Autodesk Inventor part; units mm, degrees
ref_plane "YZ Plane" through (0, 0, 0) normal (1, 0, 0) x (0, 1, 0)
ref_plane "XZ Plane" through (0, 0, 0) normal (0, 1, 0) x (-1, 0, 0)
ref_plane "XY Plane" through (0, 0, 0) normal (0, 0, 1) x (1, 0, 0)
sketch "Sketch1" plane through (0, 0, 0) normal (0, 1, 0) x (-1, 0, 0)
  arc A0 (-31.1503, 12.1688) -> (-35.4003, 7.9188) centre (-35.4003, 12.1688) ccw
  line L0 (-35.4003, 16.4188) -> (-35.4003, -2.5812)
  line L1 (-39.6503, 12.1688) -> (-31.1503, 12.1688)
  line L2 (-39.6503, -2.5812) -> (-39.6503, 12.1688)
  line L3 (-35.4003, 12.1688) -> (-26.4003, 12.1688)
  line L4 (-35.4003, 16.4188) -> (-26.4003, 16.4188)
  line L5 (-26.4003, 16.4188) -> (-26.4003, 7.9188)
  line L6 (-26.4003, 7.9188) -> (-35.4003, 7.9188)
  line L7 (-35.4003, 7.9188) -> (-35.4003, 16.4188)
  arc A1 (-35.4003, 7.9188) -> (-31.1503, 12.1688) centre (-35.4003, 12.1688) ccw
  line L8 (-35.4003, -2.5812) -> (-39.6503, -2.5812)
  point P0 (0, 0)
  dimension "d0" = 8.5
  dimension "d3" = 19
  dimension "d4" = 9
extrude "Extrusion2" add sketch "Sketch1" along normal blind 3
extrude "Extrusion3" add sketch "Sketch1" along normal blind 9 contours L1 L0 A0 | A1 L0 L1 | L0 L1 A0 | L0 A0 L1
sketch "Sketch2" plane through (35.4003, 9, 12.1688) normal (0, 1, 0) x (1, 0, 0)
  circle A0 centre (0, 0) radius 4.25
  circle A1 centre (0, 0) radius 4.25
  point P0 (-35.4003, 12.1688)
hole "Hole1" at (35.4003, 9, 12.1688) direction (0, -1, 0) diameter 2.4384 end through all
mirror "Mirror1" about plane through (39.6503, 0, -2.5812) normal (0, 0, -1) of "Extrusion2", "Extrusion3", "Hole1"
mirror "Mirror2" about plane through (26.4003, 0, -13.0812) normal (-1, 0, 0) of "Extrusion2", "Extrusion3", "Hole1", "Mirror1"
properties part number "Spacer"
Verification items for the finished model (mm, model axes). A direction names the side the tool comes from. Coordinates: 2 decimals unless noted, no trailing zeros. Order: outer loops, then holes, each group sorted by start corner. A loop starts at its lowest first (then second) coordinate and runs counter-clockwise, first axis right, second up. Notation, with made-up numbers: M 44,-28.75 L 88,-28.75 A32 cw 88,10.25 Z; hole C 58,21.5 d10. An arc over 180 degrees is marked long. One line per item, written item: value. Start each with the question number.
Item 1: Sectioned sample at C-C (x = 24). Enter the section's corners in (y, z).
Item 2: Gauge pin test, flat ends, axial feed: pin 1 (3 mm diameter, centred on x = 33.5, y = 7.5, fed in from +Z); pin 2 (1.5 mm diameter, centred on y = 6.5, z = -15.5, fed in from -X); pin 3 (2 mm diameter, centred on x = 37, z = 3, fed in from +Y); pin 4 (4 mm diameter, centred on y = 5.5, z = -5, fed in from -X). Record the tip position at first contact, or that the pin passes through.
Item 3: Sectioned sample at A-A (y = 4.5). Enter the section's corners in (x, z).
Item 4: Access from +Z, -Z, +X, -X, +Y, -Y to the whole of each face (thin tool, end or side, straight path). Record for faces 5 (the cylindrical face through (38.273, 5.437, 15.301)), 6 (the flat face through (17.4, 1, -3)), 7 (the flat face through (26, 1, -21.581)).
Item 5: Scan lines: probe 1 along Z at (x, y) = (20, 1.5); probe 2 along X at (y, z) = (2.5, 0.5); probe 3 along Z at (x, y) = (36, 8). Record each from-to range of solid material in increasing order.
Item 6: Sectioned sample at D-D (y = 2.25). Enter the section's corners in (x, z).
Item 7: Sectioned sample at B-B (z = 0). Enter the section's corners in (x, y).
Item 8: Mould release check, pull along Z, two halves, no side actions. Record for faces 1 (the flat face through (35.4, 1, -2)), 2 (the flat face through (39.65, 1, -3)), 3 (the cylindrical face through (16.19, 4.44, 12.01)), 4 (the flat face through (27, 1, 16.419)): released by +Z, released by -Z, zero draft, split by the parting line, or undercut.
Conclusion:
1. outline: M 0,-21.58 L 3,-21.58 L 3,-13.08 L 0,-13.08 Z; M 0,7.92 L 3,7.92 L 3,16.42 L 0,16.42 Z
2. pin 1: stops at z = 16.4
2. pin 2: stops at x = 13.29
2. pin 3: stops at y = 3
2. pin 4: passes through
3. outline: C 17.4,-17.33 d8.5; C 17.4,12.17 d8.5; C 35.4,-17.33 d8.5; C 35.4,12.17 d8.5; hole C 17.4,-17.33 d2.44; hole C 17.4,12.17 d2.44; hole C 35.4,-17.33 d2.44; hole C 35.4,12.17 d2.44
4. face 5: +Y
4. face 6: +Y, -Y
4. face 7: -Z, +X, -X, +Y, -Y
5. probe 1: z = -21.58 to -13.08, 7.92 to 16.42
5. probe 2: x = 13.15 to 17.4, 35.4 to 39.65
5. probe 3: z = -21.54 to -18.39, -16.27 to -13.12, 7.96 to 11.11, 13.23 to 16.38
6. outline: M 13.15,-17.33 A4.25 ccw 17.4,-21.58 L 35.4,-21.58 A4.25 ccw 39.65,-17.33 L 39.65,12.17 A4.25 ccw 35.4,16.42 L 17.4,16.42 A4.25 ccw 13.15,12.17 Z; hole C 17.4,-17.33 d2.44; hole C 17.4,12.17 d2.44; hole M 17.4,-13.08 L 35.4,-13.08 L 35.4,7.92 L 17.4,7.92 Z; hole C 35.4,-17.33 d2.44; hole C 35.4,12.17 d2.44
7. outline: M 13.15,0 L 17.4,0 L 17.4,3 L 13.15,3 Z; M 35.4,0 L 39.65,0 L 39.65,3 L 35.4,3 Z
8. face 1: undercut
8. face 2: zero draft
8. face 3: undercut
8. face 4: released by +Z
